```python
from build123d import *

# Parameters (mm, degrees)
PAD_DEPTH       = 20.2
PAD_TAPER       = -7.3
POCKET_DEPTH    = 20.2
THICKNESS_T     = -1
POCKET001_DEPTH = 1
POCKET002_DEPTH = 1
POCKET003_DEPTH = 15


with BuildPart() as part:
    # Sketch → Pad (new body)
    with BuildSketch(Plane.XZ):
        Polygon((-30.5, -30.5), (-30.5, 30.5), (30.5, 30.5), (30.5, 11.5), (-11.5, 11.5), (-11.5, -30.5), align=None)
    extrude(amount=-PAD_DEPTH, taper=PAD_TAPER)

    # Sketch001 (on Face7 of Pad) → Pocket (cut)
    with BuildSketch(Plane.XZ):
        Polygon((-30.5, -30.5), (-11.5, -30.5), (-11.5, 11.5), (30.5, 11.5), (30.5, 30.5), (30.5, 40.5), (40.5, 40.5), (40.5, -40.5), (-40.5, -40.5), (-40.5, -30.5), align=None)
    extrude(amount=-POCKET_DEPTH, mode=Mode.SUBTRACT)

    # Thickness
    thickness_openings = [part.faces().sort_by_distance(p)[0] for p in [
        (-32.188414, 20.2, 1.29384),
    ]]
    offset(amount=THICKNESS_T, openings=thickness_openings, kind=Kind.INTERSECTION)

    # Sketch002 (on Face2 of Thickness) → Pocket001 (cut)
    with BuildSketch(Plane(origin=(0, 0, -30.5), x_dir=(1, 0, 0), z_dir=(0, 0, -1))):
        Polygon((-32.08768, -20.2), (-29.628103, -1), (-12.5, -1), (-12.5, -20.2), align=None)
    extrude(amount=-POCKET001_DEPTH, mode=Mode.SUBTRACT)

    # Sketch003 (on Face6 of Thickness) → Pocket002 (cut)
    with BuildSketch(Plane.YZ.offset(30.5)):
        Polygon((20.2, 32.08768), (1, 29.628103), (1, 12.5), (20.2, 12.5), align=None)
    extrude(amount=-POCKET002_DEPTH, mode=Mode.SUBTRACT)

    # Pocket002 Face9 → Pocket003 (cut)
    with BuildSketch(Plane(origin=(-1.376471, 20.2, 1.376471), x_dir=(1, 0, 0), z_dir=(0, 1, 0))):
        Polygon((31.876471, -11.123529), (31.876471, -10.123529), (-10.123529, -10.123529), (-10.123529, 31.876471), (-11.123529, 31.876471), (-11.123529, 30.876471), (-11.123529, -11.123529), (30.876471, -11.123529), align=None)
    extrude(amount=-POCKET003_DEPTH, mode=Mode.SUBTRACT)


solid = part.part
```
CAD build for the part. Positions are in the model's coordinates, mm. A direction names the side the tool comes from. Round coordinates to 2 decimals unless told otherwise and drop trailing zeros. Return JSON: item names as keys, results as strings. Group by question number.
(1) Mould opens along X. For faces 4 (the flat face through (-30.875, 10.734, -30.007)), 5 (the flat face through (-30.867, 10.734, 0.859)), 6 (the flat face through (-1.721, 10.734, 30.867)), 7 (the flat face through (-11.5, 3, -10)) say: +X half, -X half, draft (parallel to the pull), parting line (faces both ways), or undercut.
(2) Drop flat-ended pins along their axis: P1, Ø3, axis at x = 8.5, y = 3.5, coming from the +Z side; P2, Ø3, axis at y = 16.5, z = -2.5, coming from the -X side; P3, Ø5.5, axis at y = 1.5, z = -16, coming from the +X side. Give the stop position or say it passes through.
(3) Tool access for faces 1 (the flat face through (9, 3, 11.5)), 2 (the flat face through (-12.5, 3, -9)), 3 (the flat face through (9, 3, 12.5)): list every direction of +Z, -Z, +X, -X, +Y, -Y with a clear straight run to the whole face (end or side of a thin tool).
(4) Wall check: probe 1 along Y at (x, z) = (-29.5, 3.5); probe 2 along X at (y, z) = (3.5, -6.5); probe 3 along X at (y, z) = (4.75, -0.5). Give the ranges that are in metal, low to high. Write a range as [from, to].
Answer list:
{
 "1": {"face 4": "undercut", "face 5": "undercut", "face 6": "draft", "face 7": "+X half"},
 "2": {"P1": "z = 31.14", "P2": "x = -32.81", "P3": "x = -11.5"},
 "3": {"face 1": "-Z, +X, +Y, -Y", "face 2": "-Z, +Y", "face 3": "+X, +Y"},
 "4": {"probe 1": "[0, 1]", "probe 2": "[-30.95, -29.94], [-12.5, -11.5]", "probe 3": "[-31.11, -30.1], [-12.5, -11.5]"}
}
